The figure shows three views and two pictorial views of one solid part (mm, origin at its lowest corner). Answer the questions. A direction names the side the tool comes from. Coordinates: 2 decimals unless noted, no trailing zeros. Loops run counter-clockwise (first coordinate to the right, second up) from the corner with the lowest first, then second, coordinate; pieces in that order, holes last. Notation, with made-up numbers: M 59,83 L 112,83 A10 cw 112,101 Z; hole C 28.5,-13 d7. An arc over 180 degrees is marked long. One line per item, written item: value. Start each with the question number.
1. Determine the mould class of the marked faces 6, 7, 8 and 9 for opening direction X: +X half, -X half, draft (parallel to the pull), parting line (faces both ways), or undercut.
2. Consider probe 1 along X at (y, z) = (29, 39); probe 2 along X at (y, z) = (42, 19); probe 3 along Y at (x, z) = (16.5, 35.5). Determine where each line is inside the solid, lowest interval first.
3. The part is cut by section B-B (x = 8.25). Write down the section's boundary in (y, z) (1 decimal).
4. The part is cut by section A-A (y = 10). State how many separate pieces and enclosed holes the cut face has, then the cut area to 3 significant figures.
5. The part is cut by section C-C (z = 51). Write down the section's boundary in (x, y) (1 decimal).
6. For the marked faces 1, 2, 3, 4 and 5, determine the directions among +Z, -Z, +X, -X, +Y, -Y from which every point of the face is accessible in a straight line to the end or side of a thin tool.
7. Flat-ended cylindrical pins translate along their axes: pin 1 (5.5 mm diameter, centred on y = 10, z = 5.87, fed in from +X); pin 2 (2 mm diameter, centred on x = 11.5, y = 40.5, fed in from -Z) (3 decimals); pin 3 (10 mm diameter, centred on x = 23, z = 38, fed in from -Y). Find the tip coordinate at first contact, or state that the pin passes through.
8. The part is cut by section D-D (y = 40). Write down the section's boundary in (x, z) (1 decimal), then the cut area to 3 significant figures.
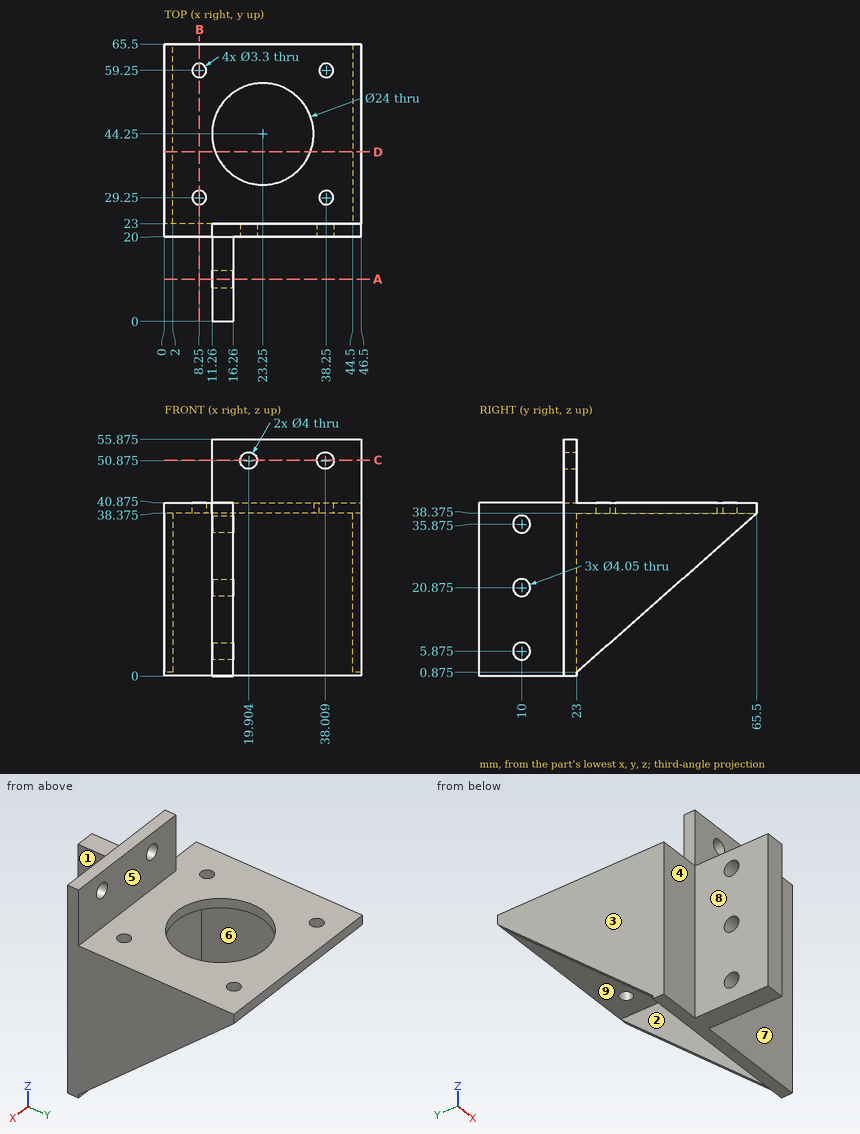
Answer block:
1. face 6: undercut
1. face 7: draft
1. face 8: -X half
1. face 9: undercut
2. probe 1: x = 0 to 6.62, 9.88 to 36.62, 39.88 to 46.5
2. probe 2: x = 0 to 2, 44.5 to 46.5
2. probe 3: y = 20 to 23
3. outline: M 20,0 L 23,0 L 23,38.4 L 27.6,38.4 L 27.6,40.9 L 20,40.9 Z; M 30.9,38.4 L 57.6,38.4 L 57.6,40.9 L 30.9,40.9 Z; M 60.9,38.4 L 65.5,38.4 L 65.5,40.9 L 60.9,40.9 Z
4. separate pieces: 4
4. enclosed holes: 0
4. area: 144 mm2
5. outline: M 11.3,20 L 17.9,20 L 17.9,23 L 11.3,23 Z; M 21.9,20 L 36,20 L 36,23 L 21.9,23 Z; M 40,20 L 46.5,20 L 46.5,23 L 40,23 Z
6. face 1: +Z, -Z, +X, -Y
6. face 2: -Z, +Y
6. face 3: +Z, -Z, -X, +Y, -Y
6. face 4: +Z, -Z, -X, -Y
6. face 5: +Z, +X, -X, +Y
7. pin 1: stops at x = 16.26
7. pin 2: stops at z = 38.375
7. pin 3: stops at y = 20
8. outline: M 0,15.9 L 2,15.9 L 2,38.4 L 12,38.4 L 12,40.9 L 0,40.9 Z; M 34.5,38.4 L 44.5,38.4 L 44.5,15.9 L 46.5,15.9 L 46.5,40.9 L 34.5,40.9 Z
8. area: 150 mm2
